Geometry check sheet. Reference: the model listing, model coordinates, mm. Coordinates: 2 decimals unless noted, no trailing zeros. Write each loop counter-clockwise with the first axis right and the second up, starting at its lowest first coordinate (ties: lowest second). Pieces come first, ordered by that corner, then holes. Notation, with made-up numbers: (79.5, 17.25) -> (109.5, 17.25) arc R32 ccw to (109.5, 51.25) -> close; hole circle Ø3 at (37.25, 23). An arc over 180 degrees is marked (long way). Answer in a Markdown table with one row per item. Add a question column.
1. Cross-section at A-A on x = 2.5. Record the cut outline in (y, z) (3 decimals), and give its area (3 significant figures).
2. Cross-section at D-D on x = 35. Record the cut outline in (y, z) (3 decimals).
3. Cross-section at B-B on y = 1.9. Record the cut outline in (x, z) (3 decimals).
4. Depth check by flat-ended pin: P1, Ø4, axis at x = 35, z = 3, coming from the +Y side (3 decimals). Enter the tip coordinate at first touch or a pass-through.
5. Cross-section at C-C on z = 3. Record the cut outline in (x, y) (3 decimals).
6. Scan lines: L1, parallel to X at y = 1.7, z = 3; L2, parallel to X at y = 0.4, z = 37.5; L3, parallel to Z at x = 2, y = 2.6. Record each from-to range of solid material in increasing order. Write a range as from..to.
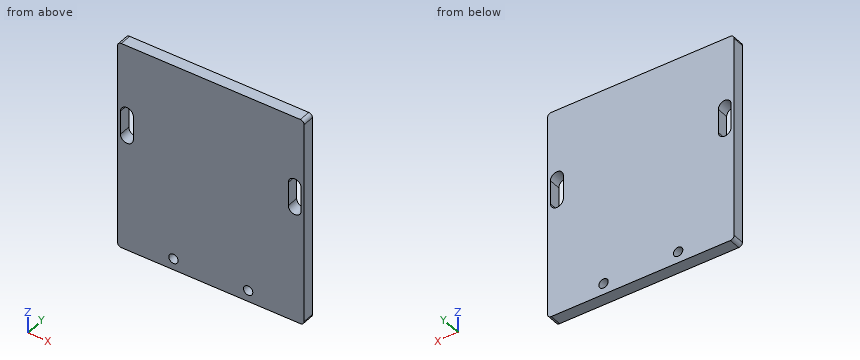
```python
from build123d import *

# Parameters (mm, degrees)
SKETCH1_W               = 50
SKETCH1_H               = 56
SKETCH1_R               = 1.1
BOSS_EXTRUDE1_DEPTH     = 3.175
FILLET1_R               = 1
M3X0_5_TAPPED_HOLE1_D   = 2.5
CUT_EXTRUDE1_DEPTH      = 76.140406074
CUT_EXTRUDE1_DEPTH_BACK = 76.140406074


with BuildPart() as part:
    # Sketch1 → Boss-Extrude1 (new body)
    with BuildSketch(Plane(origin=(0, 0, 0), x_dir=(1, 0, 0), z_dir=(0, 1, 0))):
        with Locations((25, -28)):
            Rectangle(SKETCH1_W, SKETCH1_H)
        with Locations(Location((15, -3, 0), (0, 0, 270))):
            Circle(SKETCH1_R, mode=Mode.SUBTRACT)
        with Locations(Location((35, -3, 0), (0, 0, 270))):
            Circle(SKETCH1_R, mode=Mode.SUBTRACT)
    extrude(amount=BOSS_EXTRUDE1_DEPTH)

    # Fillet1
    fillet1_edges = [part.edges().sort_by_distance(p)[0] for p in [
        (0, 1.5875, 0),
        (50, 1.5875, 0),
        (50, 1.5875, 56),
        (0, 1.5875, 56),
    ]]
    fillet(fillet1_edges, radius=FILLET1_R)

    # M3x0.5 Tapped Hole1 (through all)
    with Locations(Plane(origin=(15, 3.175, 3), x_dir=(0, 0, 1), z_dir=(0, 1, 0))):
        with Locations((0, 0), (0, 20)):
            Hole(M3X0_5_TAPPED_HOLE1_D / 2)

    # Sketch3 → Cut-Extrude1 (cut, two sides: drawn at the far end of the back side and taken through both)
    with BuildSketch(Plane(origin=(0, 3.175, 0), x_dir=(1, 0, 0), z_dir=(0, 1, 0)).offset(-CUT_EXTRUDE1_DEPTH_BACK)):
        with BuildLine():
            Line((0.775, -31), (0.775, -37.35))
            ThreePointArc((0.775, -37.35), (2.5, -39.075), (4.225, -37.35))
            Line((4.225, -37.35), (4.225, -31))
            ThreePointArc((4.225, -31), (2.5, -29.275), (0.775, -31))
        make_face()
        with BuildLine():
            Line((45.775, -31), (45.775, -37.35))
            ThreePointArc((45.775, -37.35), (47.5, -39.075), (49.225, -37.35))
            Line((49.225, -37.35), (49.225, -31))
            ThreePointArc((49.225, -31), (47.5, -29.275), (45.775, -31))
        make_face()
    extrude(amount=CUT_EXTRUDE1_DEPTH + CUT_EXTRUDE1_DEPTH_BACK, mode=Mode.SUBTRACT)


solid = part.part
```
Results found:
| question | item | result |
|---|---|---|
| 1 | outline | (0, 0) -> (3.175, 0) -> (3.175, 29.275) -> (0, 29.275) -> close; (0, 39.075) -> (3.175, 39.075) -> (3.175, 56) -> (0, 56) -> close |
| 1 | area | 147 mm^2 |
| 2 | outline | (0, 0) -> (3.175, 0) -> (3.175, 1.75) -> (0, 1.75) -> close; (0, 4.25) -> (3.175, 4.25) -> (3.175, 56) -> (0, 56) -> close |
| 3 | outline | (0, 1) arc R1 ccw to (1, 0) -> (49, 0) arc R1 ccw to (50, 1) -> (50, 55) arc R1 ccw to (49, 56) -> (1, 56) arc R1 ccw to (0, 55) -> close; hole (0.775, 31) arc R1.725 ccw to (4.225, 31) -> (4.225, 37.35) arc R1.725 ccw to (0.775, 37.35) -> close; hole circle Ø2.5 at (15, 3); hole circle Ø2.5 at (35, 3); hole (45.775, 31) arc R1.725 ccw to (49.225, 31) -> (49.225, 37.35) arc R1.725 ccw to (45.775, 37.35) -> close |
| 4 | P1 | stops at y = 3.175 |
| 5 | outline | (0, 0) -> (13.75, 0) -> (13.75, 3.175) -> (0, 3.175) -> close; (16.25, 0) -> (33.75, 0) -> (33.75, 3.175) -> (16.25, 3.175) -> close; (36.25, 0) -> (50, 0) -> (50, 3.175) -> (36.25, 3.175) -> close |
| 6 | L1 | x = 0..13.75, 16.25..33.75, 36.25..50 |
| 6 | L2 | x = 0..0.78, 4.22..45.78, 49.22..50 |
| 6 | L3 | z = 0..29.35, 39..56 |
